from build123d import *

# Parameters (mm, degrees)
SKIZZE2_W                       = 8
SKIZZE2_H                       = 22
SCHNITT_LINEAR_AUSTRAGEN1_DEPTH = 10


with BuildPart() as part:
    # Skizze1 → Rotation2 (revolve)
    with BuildSketch(Plane(origin=(0, 0, 0), x_dir=(1, 0, 0), z_dir=(0, 1, 0))):
        Polygon((0, 0), (22.902, 0), (22.902, -7), (20.902, -7), (20.902, -2), (0, -2), align=None)
    revolve(axis=Axis((0, 0, 2), (0, 0, -1)))

    # Skizze2 → Schnitt-Linear austragen1 (cut)
    with BuildSketch(Plane(origin=(0, 0, 0), x_dir=(-1, 0, 0), z_dir=(0, 0, -1))):
        Rectangle(SKIZZE2_W, SKIZZE2_H)
    extrude(amount=-SCHNITT_LINEAR_AUSTRAGEN1_DEPTH, mode=Mode.SUBTRACT)


solid = part.part
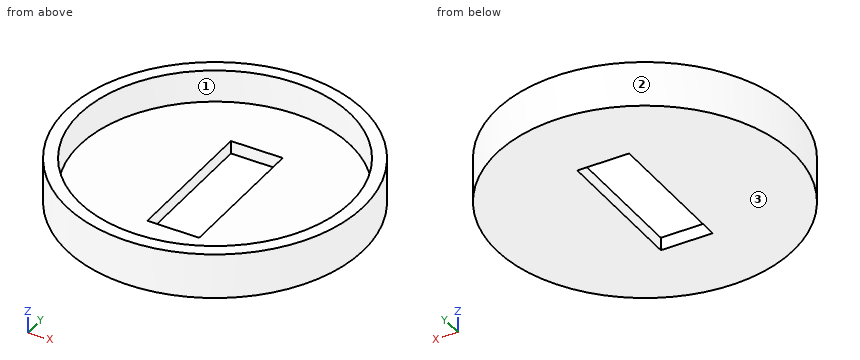
Could you check a few things on this model? Use its own coordinates, in mm. Face numbers are marked on the shaded views. Give positions to 0.01 mm unless a question says otherwise; leave off trailing zeros. Order: outer loops, then holes, each group sorted by start corner. A loop starts at its lowest first (then second) coordinate and runs counter-clockwise, first axis right, second up. Notation, with made-up numbers: (44.5, 29.25) - (89.5, 29.25) arc R28 cw to (89.5, 62.25) - close; hole circle Ø4 at (47.5, -18.5). An arc over 180 degrees is marked (long way). One line per item, written item: value. Start each with the question number.
1. Imagine slicing it at D-D on x = -10. List the corners of the cut face in (y, z) for me.
2. Imagine slicing it at B-B on y = 0. List the corners of the cut face in (x, z) for me.
3. If I drill on probe 1 along Y at (x, z) = (0, 4.1); probe 2 along X at (y, z) = (-10, 2.5), over which ranges is the centre line in solid material (lowest first)?
4. Imagine slicing it at A-A on x = 0. List the corners of the cut face in (y, z) for me.
5. Imagine slicing it at C-C on z = 1.25. List the corners of the cut face in (x, y) for me.
6. For P1, Ø0.6, axis at x = -1.5, z = 1, coming from the +Y side; P2, Ø1.5, axis at y = 11, z = 1.5, coming from the -X side; P3, Ø1.6, axis at x = 0.5, z = 1.5, coming from the -Y side, each with a flat end and sliding along its axis, tell me the tip position at first contact or that it passes through.
7. Thinking about a two-plate mould opening in X: for the marked faces 1, 2 and 3, which applies, +X half, -X half, draft (parallel to the pull), parting line (faces both ways), or undercut?
Values:
1. outline: (-20.6, 0) - (20.6, 0) - (20.6, 7) - (18.35, 7) - (18.35, 2) - (-18.35, 2) - (-18.35, 7) - (-20.6, 7) - close
2. outline: (-22.9, 0) - (-4, 0) - (-4, 2) - (-20.9, 2) - (-20.9, 7) - (-22.9, 7) - close; (4, 0) - (22.9, 0) - (22.9, 7) - (20.9, 7) - (20.9, 2) - (4, 2) - close
3. probe 1: -22.9 to -20.9, 20.9 to 22.9
3. probe 2: -20.6 to -18.35, 18.35 to 20.6
4. outline: (-22.9, 0) - (-11, 0) - (-11, 2) - (-20.9, 2) - (-20.9, 7) - (-22.9, 7) - close; (11, 0) - (22.9, 0) - (22.9, 7) - (20.9, 7) - (20.9, 2) - (11, 2) - close
5. outline: circle Ø45.8 at (0, 0); hole (-4, -11) - (4, -11) - (4, 11) - (-4, 11) - close
6. P1: y = 22.87
6. P2: x = -20.48
6. P3: y = -22.9
7. face 1: undercut
7. face 2: parting line
7. face 3: draft
